The model under review builds one solid part; all positions refer to its coordinate system, in mm. Face numbers are marked on the shaded views. A direction names the side the tool comes from. Coordinates: 2 decimals unless noted, no trailing zeros. Write each loop counter-clockwise with the first axis right and the second up, starting at its lowest first coordinate (ties: lowest second). Pieces come first, ordered by that corner, then holes. Notation, with made-up numbers: (-24.5, -13.5) -> (9.5, -13.5) arc R17 cw to (9.5, 8.5) -> close; hole circle Ø2 at (76.5, -17.75). An arc over 180 degrees is marked (long way). Put each result on its own line as item: value. Start each with the question number.
Autodesk Fusion 360 part; units mm, degrees
sketch "Sketch1" plane through (0, 0, 0) normal (0, 1, 0) x (1, 0, 0)
  line L0 (0, 0) -> (80, 0)
  line L1 (80, 0) -> (80, 80)
  line L2 (80, 80) -> (0, 80)
  line L3 (0, 80) -> (0, 0)
  circle A0 centre (40, 40) radius 15
  line L4 (0, 20) -> (20, 0)
  dimension "d1" = 80
  dimension "d2" = 80
  dimension "d3" = 30
  dimension "d4" = 40
  dimension "d5" = 40
  dimension "d6" = 20
  dimension "d7" = 20
extrude "Extrude1" add sketch "Sketch1" along normal blind 10 contours L0 L1 L2 L3 L4
sketch "Sketch2" plane through (0, 10, 0) normal (0, 1, 0) x (-1, 0, 0)
  circle A0 centre (-40, -40) radius 15
  line L0 (0, -20) -> (-20, 0)
  line L1 (-20, 0) -> (-80, 0)
  line L2 (-80, 0) -> (-80, -80)
  line L3 (-80, -80) -> (0, -80)
  line L4 (0, -80) -> (0, -20)
  line L5 (0, -80) -> (-80, -80)
  line L6 (-80, -80) -> (-80, -70)
  line L7 (-80, -70) -> (0, -70)
  line L8 (0, -70) -> (0, -80)
  line L9 (-80, -80) -> (-70, -80)
  line L10 (-70, -80) -> (-70, 0)
  line L11 (-70, 0) -> (-80, 0)
  line L12 (-80, 0) -> (-80, -80)
  dimension "d10" = 10
  dimension "d11" = 10
extrude "Extrude2" add sketch "Sketch2" along normal blind 40 contours L3 L4 L5 L7 L8 L10 | L1 L2 L7 L10 L11 L12 | L2 L3 L5 L6 L7 L9 L10 L12
fillet "Fillet1" radius 5 1 edges at (70, 30, -70)
fillet "Fillet2" radius 15 1 edges at (80, 25, -80)
sketch "Sketch3" plane through (70, 0, 0) normal (-1, 0, 0) x (0, 0, 1)
  line L0 (-65, 50) -> (-65, 10)
  line L1 (-65, 10) -> (0, 10)
  line L2 (0, 10) -> (0, 50)
  line L3 (0, 50) -> (-65, 50)
  circle A0 centre (-35, 30) radius 7.5
  dimension "d18" = 15
  dimension "d19" = 35
  dimension "d20" = 20
extrude "Extrude3" cut sketch "Sketch3" against normal blind 10 contours A0
sketch "Sketch4" plane through (0, 0, -70) normal (0, 0, 1) x (1, 0, 0)
  line L0 (65, 10) -> (65, 50)
  line L1 (65, 50) -> (0, 50)
  line L2 (0, 50) -> (0, 10)
  line L3 (0, 10) -> (65, 10)
  circle A0 centre (35, 30) radius 7.5
  dimension "d23" = 15
  dimension "d24" = 35
  dimension "d25" = 20
extrude "Extrude4" cut sketch "Sketch4" against normal blind 10 contours A0
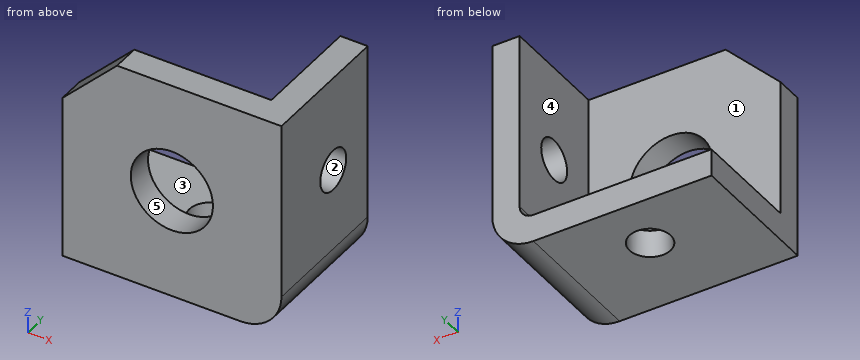
1. Consider section A-A on z = -49. State the section outline as (x, y) points, then the cut area to 3 significant figures.
2. Wall thickness on line 1 (Z direction, x = 40, y = 7); line 2 (X direction, y = 6, z = -40); line 3 (Y direction, x = 74.5, z = -35): over which ranges is each line inside the solid? List them lowest first. Write a range as from..to.
3. The part is to be moulded in two halves that separate along Z. For the marked faces 3, 4 and 5, say which applies: released by +Z, released by -Z, zero draft, split by the parting line, or undercut.
4. Tool access review of the marked faces 1 and 2: name each direction out of +Z, -Z, +X, -X, +Y, -Y from which nothing blocks a thin tool from reaching the whole face with its end or side.
5. Consider section D-D on z = -40. State the section outline as (x, y) points.
6. Consider section B-B on y = 30. State the section outline as (x, z) points, then the cut area to 3 significant figures.
7. Consider section C-C on x = 35. State the section outline as (y, z) points, then the cut area to 3 significant figures.
8. Insertion check: P1, Ø12, axis at x = 18.5, y = 5.5, coming from the +Z side; P2, Ø19.5, axis at y = 30, z = -35, coming from the -X side; P3, Ø8, axis at y = 11, z = -11, coming from the -X side; P4, Ø1.5, axis at x = 8.5, y = 25, coming from the +Z side. Each pin has a flat end and moves straight along its axis. Give the tip position at first contact, or say it passes through.
Output values:
1. outline: (0, 0) -> (28, 0) -> (28, 10) -> (0, 10) -> close; (52, 0) -> (80, 0) -> (80, 50) -> (70, 50) -> (70, 10) -> (52, 10) -> close
1. area: 960 mm^2
2. line 1: z = -80..-55, -25..0
2. line 2: x = 0..25, 55..80
2. line 3: y = 0..22.5, 37.5..50
3. face 3: released by +Z
3. face 4: zero draft
3. face 5: undercut
4. face 1: +Z, -X, +Y
4. face 2: +X, -X
5. outline: (0, 0) -> (25, 0) -> (25, 10) -> (0, 10) -> close; (55, 0) -> (80, 0) -> (80, 24.41) -> (70, 24.41) -> (70, 10) -> (55, 10) -> close; (70, 35.59) -> (80, 35.59) -> (80, 50) -> (70, 50) -> close
6. outline: (0, -80) -> (27.5, -80) -> (27.5, -70) -> (0, -70) -> close; (42.5, -80) -> (65, -80) arc R15 ccw to (80, -65) -> (80, -42.5) -> (70, -42.5) -> (70, -65) arc R5 cw to (65, -70) -> (42.5, -70) -> close; (70, -27.5) -> (80, -27.5) -> (80, 0) -> (70, 0) -> close
6. area: 1,160 mm^2
7. outline: (0, -80) -> (22.5, -80) -> (22.5, -70) -> (10, -70) -> (10, -54.14) -> (0, -54.14) -> close; (0, -25.86) -> (10, -25.86) -> (10, 0) -> (0, 0) -> close; (37.5, -80) -> (50, -80) -> (50, -70) -> (37.5, -70) -> close
7. area: 767 mm^2
8. P1: stops at z = 0
8. P2: stops at x = 70
8. P3: stops at x = 5.13
8. P4: stops at z = -70
